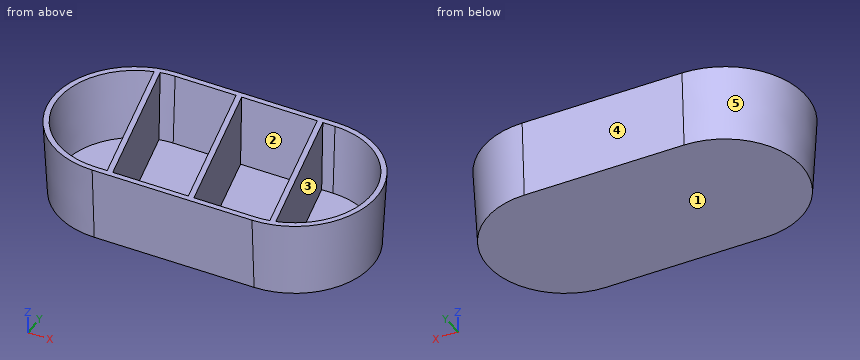
from build123d import *

# Parameters (mm, degrees)
F1_DEPTH = 14
F1_TAPER = 3
F2_T     = -1
F4_DEPTH = 13


with BuildPart() as f1:
    # F0 (on Top) → F1 (new body)
    with BuildSketch(Plane.XY):
        with BuildLine():
            Line((14.5999998801, 14.9), (-14.6000001199, 14.9))
            ThreePointArc((-14.6000001199, 14.9), (-29.5000001199, 0), (-14.6000001199, -14.9))
            Line((-14.6000001199, -14.9), (14.6000003597, -14.9))
            ThreePointArc((14.6000003597, -14.9), (29.4999998801, 2.398e-07), (14.5999998801, 14.9))
        make_face()
    extrude(amount=-F1_DEPTH, taper=F1_TAPER)

    # F2
    f2_openings = [f1.faces().sort_by_distance(p)[0] for p in [
        (0, 0, 0),
    ]]
    offset(amount=F2_T, openings=f2_openings)

    # F3 (on face) → F4 (join, through all)
    with BuildSketch(Plane.XY.offset(-13)):
        Polygon((-2.4430742086, 13.898627654), (-3.4654148035, 13.898627654), (2.4430742086, -13.898627654), (3.4654148035, -13.898627654), align=None)
        with BuildLine():
            ThreePointArc((-17.2142812839, 13.6505452148), (-17.7037250021, 13.5476471212), (-18.1891496276, 13.4272058328))
            Line((-18.1891496276, 13.4272058328), (-12.3808644169, -13.898627654))
            Line((-12.3808644169, -13.898627654), (-11.358523822, -13.898627654))
            Line((-11.358523822, -13.898627654), (-17.2142812839, 13.6505452148))
        make_face()
        with BuildLine():
            Line((12.3808644169, 13.898627654), (11.358523822, 13.898627654))
            Line((11.358523822, 13.898627654), (17.2142812745, -13.6505451706))
            ThreePointArc((17.2142812745, -13.6505451706), (17.7037249911, -13.5476470688), (18.1891496147, -13.4272057721))
            Line((18.1891496147, -13.4272057721), (12.3808644169, 13.898627654))
        make_face()
    extrude(amount=F4_DEPTH)


solid = f1.part
Here's how the part is built. I have some questions about the finished solid (model axes, mm). Face numbers are marked on the shaded views. A direction names the side the tool comes from. Round coordinates to 2 decimals unless told otherwise and drop trailing zeros. Return JSON: item names as keys, results as strings.
Q1. Which directions (+Z, -Z, +X, -X, +Y, -Y) give clear straight access to the entire face, cutting with the end or side of a thin tool? Please do the marked faces 1 and 2.
Filled sheet:
{"face 1": "-Z, +X, -X, +Y, -Y", "face 2": "+Z"}
Q2. If we mould it in two halves opening along X, with no side actions, what happens to the marked faces 3, 4 and 5? For each: released by +X, released by -X, zero draft, split by the parting line, or undercut.
Filled sheet:
{"face 3": "undercut", "face 4": "zero draft", "face 5": "released by -X"}
Q3. If we section it at A-A on z = -11.75: Give the number of separate pieces and of enclosed holes in the cut face, plus the area to 3 significant figures.
Filled sheet:
{"separate pieces": "1", "enclosed holes": "4", "area": "226 mm^2"}
Q4. For pin 1 Ø9.5 at (x, y) = (3.5, -6) entering from +Z; pin 2 Ø8 at (x, z) = (-1.5, -12) entering from -Y; pin 3 Ø4 at (y, z) = (2.5, -12) entering from -X; pin 4 Ø6 at (y, z) = (-4.5, -3) entering from +X, each with a flat end and sliding along its axis, tell me the tip position at first contact or that it passes through.
Filled sheet:
{"pin 1": "stops at z = 0", "pin 2": "stops at y = -14.48", "pin 3": "stops at x = -28.91", "pin 4": "stops at x = 29.3"}
Q5. I need wall thicknesses on line 1 along X through (y, z) = (-0.5, -0.75); line 2 along X through (y, z) = (11.5, -2.75); line 3 along Z through (x, y) = (24, -3). Which ranges of each line are inside material? Lowest first, please. Write a range as from..to.
Filled sheet:
{"line 1": "x = -29.45..-28.45, -15.23..-14.21, -0.4..0.62, 14.42..15.44, 28.45..29.45", "line 2": "x = -23.85..-22.15, -17.78..-16.76, -2.96..-1.93, 11.87..12.89, 22.15..23.85", "line 3": "z = -14..-13"}
